from build123d import *

# Parameters (mm, degrees)
BOSS_EXTRUDE1_DEPTH     = 27.94
CUT_EXTRUDE1_DEPTH      = 17.78
CUT_EXTRUDE1_DEPTH_BACK = 17.78
SKETCH2_R               = 1.5
SKETCH2_R_2             = 1.554918768
SKETCH2_R_3             = 1.519223358
SKETCH2_3_R             = 1.8175
SKETCH2_3_R_2           = 1.5
SKETCH2_3_R_3           = 1.872418768
SKETCH2_3_R_4           = 1.554918768
SKETCH2_3_R_5           = 1.836723358
SKETCH2_3_R_6           = 1.519223358
CUT_EXTRUDE2_DEPTH      = 17.78
BOSS_EXTRUDE2_START     = -0.7112
BOSS_EXTRUDE2_DEPTH     = 0.7112


with BuildPart() as part:
    # Sketch1 → Boss-Extrude1 (new body)
    with BuildSketch(Plane(origin=(0, 0, 0), x_dir=(1, 0, 0), z_dir=(0, 1, 0))):
        with BuildLine():
            Line((70.498234913, 37.451765087), (69.331862428, 31.209804239))
            ThreePointArc((69.331862428, 31.209804239), (72.423610275, 30.470176889), (75.425897806, 29.425082184))
            ThreePointArc((75.425897806, 29.425082184), (95.114662615, -2.928413856), (69.818170226, -31.115))
            ThreePointArc((69.818170226, -31.115), (66.675, -31.590851128), (63.5, -31.75))
            Line((63.5, -31.75), (63.5, -38.1))
            ThreePointArc((63.5, -38.1), (101.437595139, -3.514096627), (70.498234913, 37.451765087))
        make_face()
    extrude(amount=BOSS_EXTRUDE1_DEPTH)

    # Sketch2 → Cut-Extrude1 (cut, two sides: drawn at the far end of the back side and taken through both)
    with BuildSketch(Plane.ZY.offset(-63.5).offset(-CUT_EXTRUDE1_DEPTH_BACK)):
        with Locations(Location((34.821497506, 11.418652896, 0), (0, 0, 180))):
            Circle(SKETCH2_R)
        with Locations(Location((35.069922057, 3.654275356, 0), (0, 0, 180))):
            Circle(SKETCH2_R_2)
        with Locations(Location((-34.532766251, 13.194759825, 0), (0, 0, 180))):
            Circle(SKETCH2_R_3)
        with Locations(Location((-34.532766251, 3.654275356, 0), (0, 0, 180))):
            Circle(SKETCH2_R)
    extrude(amount=CUT_EXTRUDE1_DEPTH + CUT_EXTRUDE1_DEPTH_BACK, mode=Mode.SUBTRACT)

    # Sketch2_3 → Cut-Extrude2 (cut)
    # profile 1 of 4: a face of its own
    with BuildSketch(Plane.ZY.offset(-63.5)):
        with Locations((34.821497506, 11.418652896)):
            Circle(SKETCH2_3_R)
        with Locations((34.821497506, 11.418652896)):
            Circle(SKETCH2_3_R_2, mode=Mode.SUBTRACT)
    # profile 2 of 4: a face of its own
    with BuildSketch(Plane.ZY.offset(-63.5)):
        with Locations((35.069922057, 3.654275356)):
            Circle(SKETCH2_3_R_3)
        with Locations((35.069922057, 3.654275356)):
            Circle(SKETCH2_3_R_4, mode=Mode.SUBTRACT)
    # profile 3 of 4: a face of its own
    with BuildSketch(Plane.ZY.offset(-63.5)):
        with Locations((-34.532766251, 13.194759825)):
            Circle(SKETCH2_3_R_5)
        with Locations((-34.532766251, 13.194759825)):
            Circle(SKETCH2_3_R_6, mode=Mode.SUBTRACT)
    # profile 4 of 4: a face of its own
    with BuildSketch(Plane.ZY.offset(-63.5)):
        with Locations((-34.532766251, 3.654275356)):
            Circle(SKETCH2_3_R)
        with Locations((-34.532766251, 3.654275356)):
            Circle(SKETCH2_3_R_2, mode=Mode.SUBTRACT)
    extrude(amount=-CUT_EXTRUDE2_DEPTH, mode=Mode.SUBTRACT)

    # Sketch1_2 → Boss-Extrude2 (add)
    with BuildSketch(Plane(origin=(0, 0, 0), x_dir=(1, 0, 0), z_dir=(0, 1, 0)).offset(BOSS_EXTRUDE2_START)):
        with BuildLine():
            Line((70.498234913, 37.451765087), (69.331862428, 31.209804239))
            ThreePointArc((69.331862428, 31.209804239), (72.423610275, 30.470176889), (75.425897806, 29.425082184))
            ThreePointArc((75.425897806, 29.425082184), (95.114662615, -2.928413856), (69.818170226, -31.115))
            ThreePointArc((69.818170226, -31.115), (66.675, -31.590851128), (63.5, -31.75))
            Line((63.5, -31.75), (63.5, -38.1))
            ThreePointArc((63.5, -38.1), (101.437595139, -3.514096627), (70.498234913, 37.451765087))
        make_face()
    extrude(amount=BOSS_EXTRUDE2_DEPTH)


solid = part.part
Geometry check sheet. Reference: the model listing, model coordinates, mm. A direction names the side the tool comes from. Round coordinates to 2 decimals unless told otherwise and drop trailing zeros. Order: outer loops, then holes, each group sorted by start corner. A loop starts at its lowest first (then second) coordinate and runs counter-clockwise, first axis right, second up. Notation, with made-up numbers: (-26, 76.5) - (-3, 76.5) arc R16 cw to (-3, 95.5) - close; hole circle Ø11 at (37, -39.5). An arc over 180 degrees is marked (long way). One line per question, with ' | ' between items. Start each with the question number.
(1) Sectioned sample at A-A on x = 80. Record the cut outline in (y, z) (1 decimal).
(2) Sectioned sample at D-D on x = 91.5. Record the cut outline in (y, z).
(3) Sectioned sample at C-C on z = -13. Record the cut outline in (x, y).
(4) Depth check by flat-ended pin: pin 1 Ø1.1 at (y, z) = (13, -33.5) entering from -X; pin 2 Ø3 at (y, z) = (3.65, 35.07) entering from +X; pin 3 Ø4 at (x, y) = (85.5, 10) entering from -Z. Enter the tip coordinate at first touch or a pass-through.
(5) Thickness scan on L1, parallel to Z at x = 76.5, y = 2; L2, parallel to Y at x = 66, z = 34; L3, parallel to Z at x = 75.5, y = 12. Record the ranges inside material, lowest first. Write a range as [from, to].
(6) Access from +Z, -Z, +X, -X, +Y, -Y to the whole of each face (thin tool, end or side, straight path). Record for faces 1 (the flat face through (69.534, 13.414, -32.294)), 2 (the cylindrical face through (74.1, 4.2, -32.8)).
(7) Sectioned sample at B-B on y = 23. Record the cut outline in (x, z) (3 decimals).
(8) Release check for a two-part mould opening along Y. For faces 3 (the cylindrical face through (70.29, 11.499, 33.006)), 4 (the flat face through (95, 27.94, 9)), 5 (the flat face through (95, -0.711, 9)) record: released by +Y, released by -Y, zero draft, split by the parting line, or undercut.
Conclusion:
1) outline: (-0.7, -34.3) - (1.8, -34.3) arc R1.8 cw to (5.5, -34.3) - (11.4, -34.3) arc R1.8 cw to (15, -34.3) - (27.9, -34.3) - (27.9, -27.1) - (-0.7, -27.1) - close; (-0.7, 27.1) - (27.9, 27.1) - (27.9, 34.3) - (13.2, 34.3) arc R1.8 cw to (9.7, 34.3) - (5.4, 34.3) arc R1.9 cw to (1.9, 34.3) - (-0.7, 34.3) - close
2) outline: (-0.71, -25.84) - (27.94, -25.84) - (27.94, -14.97) - (-0.71, -14.97) - close; (-0.71, 14.97) - (27.94, 14.97) - (27.94, 25.84) - (-0.71, 25.84) - close
3) outline: (92.47, -0.71) - (99.31, -0.71) - (99.31, 27.94) - (92.47, 27.94) - close
4) pin 1: stops at x = 81.28 | pin 2: stops at x = 81.52 | pin 3: stops at z = -32.43
5) L1: z = [-35.81, -35.29], [-33.78, -28.97], [28.97, 34.19] | L2: y = [-0.71, 2.12], [5.19, 9.8], [13.04, 27.94] | L3: z = [-36.16, -35.93], [-33.14, -29.39], [29.39, 33.1]
6) face 1: -Z, -X, +Y, -Y | face 2: -X
7) outline: (63.5, 31.75) arc R31.75 cw to (69.332, -31.21) - (70.498, -37.452) arc R38.1 ccw to (63.5, 38.1) - close
8) face 3: undercut | face 4: released by +Y | face 5: released by -Y
